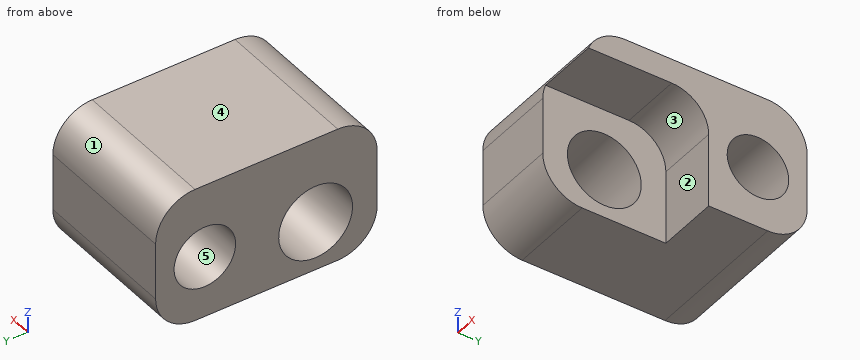
from build123d import *

# Parameters (mm, degrees)
SKETCH1_W           = 5.5
SKETCH1_H           = 9
SKETCH1_R           = 1.5
SKETCH1_R_2         = 1.25
BOSS_EXTRUDE1_DEPTH = 6
SKETCH2_W           = 4.5
SKETCH2_H           = 5
CUT_EXTRUDE1_DEPTH  = 2.5
FILLET1_R           = 1.5
FILLET2_R           = 1.6


with BuildPart() as part:
    # Sketch1 → Boss-Extrude1 (new body)
    with BuildSketch(Plane(origin=(0, 0, 0), x_dir=(0, 0, -1), z_dir=(1, 0, 0))):
        with Locations((2.75, 4.5)):
            Rectangle(SKETCH1_W, SKETCH1_H)
        with Locations((3.5, 2.5)):
            Circle(SKETCH1_R, mode=Mode.SUBTRACT)
        with Locations((3, 7)):
            Circle(SKETCH1_R_2, mode=Mode.SUBTRACT)
    extrude(amount=BOSS_EXTRUDE1_DEPTH)

    # Sketch2 → Cut-Extrude1 (cut)
    with BuildSketch(Plane(origin=(6, 0, 0), x_dir=(0, 0, -1), z_dir=(1, 0, 0))):
        with Locations((3.25, 2.5)):
            Rectangle(SKETCH2_W, SKETCH2_H)
    extrude(amount=-CUT_EXTRUDE1_DEPTH, mode=Mode.SUBTRACT)

    # Fillet1
    fillet1_edges = [part.edges().sort_by_distance(p)[0] for p in [
        (4.75, 5, -1),
    ]]
    fillet(fillet1_edges, radius=FILLET1_R)

    # Fillet2
    fillet2_edges = [part.edges().sort_by_distance(p)[0] for p in [
        (3, 9, 0),
        (3, 0, 0),
        (1.75, 0, -5.5),
        (3, 9, -5.5),
    ]]
    fillet(fillet2_edges, radius=FILLET2_R)


solid = part.part
The model under review builds one solid part; all positions refer to its coordinate system, in mm. Face numbers are marked on the shaded views. A direction names the side the tool comes from. Give positions to 0.01 mm unless a question says otherwise; leave off trailing zeros. Loops run counter-clockwise (first coordinate to the right, second up) from the corner with the lowest first, then second, coordinate; pieces in that order, holes last. Notation, with made-up numbers: (43, 87) -> (97, 87) arc R20 cw to (97, 107) -> close; hole circle Ø5 at (0, 54). An arc over 180 degrees is marked (long way). Put each result on its own line as item: value. Start each with the question number.
1. We need section B-B on x = 2.7. State the section outline as (y, z) points, then the cut area to 3 significant figures.
2. We need section A-A on y = 7. State the section outline as (x, z) points, then the cut area to 3 significant figures.
3. Wall thickness on probe 1 along Y at (x, z) = (1.5, -3.75); probe 2 along Y at (x, z) = (1.45, -3.5); probe 3 along Z at (x, y) = (1.1, 2.5): over which ranges is each line inside the solid? List them lowest first.
4. We need section D-D on x = 4.85. State the section outline as (y, z) points.
5. We need section C-C on z = -3.1. State the section outline as (x, y) points, then the cut area to 3 significant figures.
6. For the marked faces 1 and 2, list the 3-axis set-ups (+Z, -Z, +X, -X, +Y, -Y) from which the entire face can be reached by the end or side of a thin tool; tool diameter is ignored.
7. Clearance check with flat-ended pins moving along their axes: P1, Ø0.8, axis at x = 4, y = 2, coming from the -Z side; P2, Ø2, axis at y = 7, z = -3, coming from the -X side; P3, Ø0.8, axis at x = 5, z = -4.5, coming from the -Y side. State where each tip first meets the part, or that it passes through.
8. Mouldability with a two-part tool opening along Z and no side actions: class the marked faces 3, 4 and 5 as released by +Z, released by -Z, zero draft, split by the parting line, or undercut.
Determined:
1. outline: (0, -3.9) arc R1.6 ccw to (1.6, -5.5) -> (7.4, -5.5) arc R1.6 ccw to (9, -3.9) -> (9, -1.6) arc R1.6 ccw to (7.4, 0) -> (1.6, 0) arc R1.6 ccw to (0, -1.6) -> close; hole circle Ø3 at (2.5, -3.5); hole circle Ø2.5 at (7, -3)
1. area: 35.3 mm^2
2. outline: (0, -5.5) -> (6, -5.5) -> (6, -4.25) -> (0, -4.25) -> close; (0, -1.75) -> (6, -1.75) -> (6, 0) -> (0, 0) -> close
2. area: 18.0 mm^2
3. probe 1: 0 to 1.02, 3.98 to 6, 8 to 9
3. probe 2: 0 to 1, 4 to 5.85, 8.15 to 9
3. probe 3: -5.5 to -5, -2 to 0
4. outline: (0.12, -1) -> (3.5, -1) arc R1.5 cw to (5, -2.5) -> (5, -5.5) -> (7.4, -5.5) arc R1.6 ccw to (9, -3.9) -> (9, -1.6) arc R1.6 ccw to (7.4, 0) -> (1.6, 0) arc R1.6 ccw to start; hole circle Ø2.5 at (7, -3)
5. outline: (0, 0) -> (3.5, 0) -> (3.5, 1.05) -> (0, 1.05) -> close; (0, 3.95) -> (3.5, 3.95) -> (3.5, 5) -> (6, 5) -> (6, 5.75) -> (0, 5.75) -> close; (0, 8.25) -> (6, 8.25) -> (6, 9) -> (0, 9) -> close
5. area: 16.4 mm^2
6. face 1: +Z, +X, -X, +Y
6. face 2: -Z, +X, -Y
7. P1: z = -1
7. P2: through
7. P3: y = 5
8. face 3: released by -Z
8. face 4: released by +Z
8. face 5: undercut
